```python
from build123d import *

# Parameters (mm, degrees)
SKETCH1_W               = 76.2
SKETCH1_H               = 25.4
SKETCH1_W_2             = 70.104
SKETCH1_H_2             = 19.304
BOSS_EXTRUDE1_DEPTH     = 500
SKETCH3_W               = 76.2
SKETCH3_H               = 25.4
SKETCH3_W_2             = 70.104
SKETCH3_H_2             = 19.304
BOSS_EXTRUDE2_DEPTH     = 38.1
SKETCH4_W               = 76.2
SKETCH4_H               = 25.4
SKETCH4_W_2             = 70.104
SKETCH4_H_2             = 19.304
BOSS_EXTRUDE3_DEPTH     = 38.1
CUT_EXTRUDE1_DEPTH      = 13.7
CUT_EXTRUDE1_DEPTH_BACK = 13.7
CUT_EXTRUDE2_DEPTH      = 13.7
CUT_EXTRUDE2_DEPTH_BACK = 13.7


with BuildPart() as part:
    # Sketch1 → Boss-Extrude1 (new body)
    with BuildSketch(Plane(origin=(0, 0, 0), x_dir=(1, 0, 0), z_dir=(0, 1, 0))):
        Rectangle(SKETCH1_W, SKETCH1_H)
        Rectangle(SKETCH1_W_2, SKETCH1_H_2, mode=Mode.SUBTRACT)
    extrude(amount=BOSS_EXTRUDE1_DEPTH)

    # Sketch3 → Boss-Extrude2 (add)
    with BuildSketch(Plane.XZ):
        Rectangle(SKETCH3_W, SKETCH3_H)
        Rectangle(SKETCH3_W_2, SKETCH3_H_2, mode=Mode.SUBTRACT)
    extrude(amount=BOSS_EXTRUDE2_DEPTH)

    # Sketch4 → Boss-Extrude3 (add)
    with BuildSketch(Plane(origin=(0, 500, 0), x_dir=(1, 0, 0), z_dir=(0, 1, 0))):
        Rectangle(SKETCH4_W, SKETCH4_H)
        Rectangle(SKETCH4_W_2, SKETCH4_H_2, mode=Mode.SUBTRACT)
    extrude(amount=BOSS_EXTRUDE3_DEPTH)

    # Sketch5 → Cut-Extrude1 (cut, two sides)
    with BuildSketch(Plane.XY) as cut_extrude1_sk:
        Polygon((-62.772673854, 62.772673854), (63.030718061, -63.030718061), (-91.484443541, -186.384573668), (-217.287835457, -60.581181752), align=None)
    extrude(amount=CUT_EXTRUDE1_DEPTH, mode=Mode.SUBTRACT)
    extrude(cut_extrude1_sk.sketch, amount=-CUT_EXTRUDE1_DEPTH_BACK, mode=Mode.SUBTRACT)

    # Sketch6 → Cut-Extrude2 (cut, two sides)
    with BuildSketch(Plane.YX) as cut_extrude2_sk:
        Polygon((393.890988206, -106.109011794), (558.855850204, 58.855850204), (555.016088259, -106.109011794), align=None)
    extrude(amount=CUT_EXTRUDE2_DEPTH, mode=Mode.SUBTRACT)
    extrude(cut_extrude2_sk.sketch, amount=-CUT_EXTRUDE2_DEPTH_BACK, mode=Mode.SUBTRACT)


solid = part.part
```
Here's how the part is built. I have some questions about the finished solid (model axes, mm). A direction names the side the tool comes from. Coordinates: 2 decimals unless noted, no trailing zeros. Order: outer loops, then holes, each group sorted by start corner. A loop starts at its lowest first (then second) coordinate and runs counter-clockwise, first axis right, second up.
Item 1: If we section it at B-B, the plane z = -2.75: List the corners of the cut face in (x, y) for me.
Response values:
outline: (-38.1, 38.1) - (-35.05, 35.05) - (-35.05, 464.95) - (-38.1, 461.9) - close; (35.05, -35.05) - (38.1, -38.1) - (38.1, 538.1) - (35.05, 535.05) - close
Item 2: Which directions (+Z, -Z, +X, -X, +Y, -Y) give clear straight access to the entire face, cutting with the end or side of a thin tool? Please do faces 5 (the face through (-3, 3, 10)), 6 (the face through (35.052, 246, 0)).
Response values:
face 5: +Z, -Z, -X, -Y
face 6: +Y, -Y
Item 3: If we section it at D-D, the plane y = 9.5: List the corners of the cut face in (x, z) for me, then the cut area to 3 significant figures.
Response values:
outline: (-9.5, -12.7) - (38.1, -12.7) - (38.1, 12.7) - (-9.5, 12.7) - (-9.5, 9.65) - (35.05, 9.65) - (35.05, -9.65) - (-9.5, -9.65) - close
area: 349 mm2
Item 4: I need wall thicknesses on probe 1 along X at (y, z) = (459, 6.75); probe 2 along Z at (x, y) = (-20, 307); probe 3 along X at (y, z) = (511.5, 4.5). Which ranges of each line are inside material? Lowest first, please.
Response values:
probe 1: x = -38.1 to -35.05, 35.05 to 38.1
probe 2: z = -12.7 to -9.65, 9.65 to 12.7
probe 3: x = 35.05 to 38.1
Item 5: If we section it at C-C, the plane y = 397.5: List the corners of the cut face in (x, z) for me.
Response values:
outline: (-38.1, -12.7) - (38.1, -12.7) - (38.1, 12.7) - (-38.1, 12.7) - close; hole (-35.05, -9.65) - (35.05, -9.65) - (35.05, 9.65) - (-35.05, 9.65) - close
Item 6: Thinking about a two-plate mould opening in Z: for faces 1 (the face through (-1, 246, -12.7)), 2 (the face through (-38.1, 247, 0)), 3 (the face through (-35.052, 247, 0)), 4 (the face through (0, 246, 9.652)), which applies, pulls with the +Z half, pulls with the -Z half, needs draft (parallel to the pull), parting line crosses it, or undercut?
Response values:
face 1: pulls with the -Z half
face 2: needs draft
face 3: undercut
face 4: undercut
Item 7: If we section it at A-A, the plane x = 21: List the corners of the cut face in (y, z) for me, then the cut area to 3 significant figures.
Response values:
outline: (-21, -12.7) - (521, -12.7) - (521, -9.65) - (-21, -9.65) - close; (-21, 9.65) - (521, 9.65) - (521, 12.7) - (-21, 12.7) - close
area: 3,300 mm2
